Can you work these out from the model? Positions are in its coordinate system, mm. A direction names the side the tool comes from. Round coordinates to 2 decimals unless told otherwise and drop trailing zeros. Write each loop counter-clockwise with the first axis right and the second up, starting at its lowest first coordinate (ties: lowest second). Pieces come first, ordered by that corner, then holes. Notation, with made-up numbers: M 73.25,52.5 L 85.25,52.5 A19 cw 85.25,61.5 Z; hole C 75,2 d7. An arc over 180 degrees is marked long. Answer as a JSON object with one key per item and string values. Group by question number.
1) Suppose I cut it at B-B, the plane y = 3.05. Write out the boundary of the cut face in (x, z), and give its area (3 significant figures).
2) If we mould it in two halves opening along Z, with no side actions, what happens to faces 4 (the flat face through (21, 4, 24.95)), 5 (the flat face through (-44.95, 4, 0)), 6 (the cylindrical face through (-0.06, 1.02, -20.66))? For each: +Z half, -Z half, draft (parallel to the pull), parting line (faces both ways), or undercut.
3) On a 3-axis mill with a long thin cutter (end or side, diameter ignored), from which of +Z, -Z, +X, -X, +Y, -Y can I reach the whole of each face in a straight line? I mean faces 1 (the flat face through (2.65, 1.9, 25.1)), 2 (the flat face through (-38.59, 3.84, -24.126)), 3 (the flat face through (-3.5, 3.8, 24.1)). Say none if no direction works.
4) Suppose I cut it at C-C, the plane x = -27.5. Write out the boundary of the cut face in (y, z).
5) I'm going to push flat-ended pins straight in: pin 1 Ø1 at (y, z) = (3.5, 25.5) entering from -X; pin 2 Ø1 at (y, z) = (1.5, -25.5) entering from +X; pin 3 Ø2.5 at (y, z) = (3, 24.5) entering from -X; pin 4 Ø10 at (x, z) = (-10, 0.5) entering from -Y. Where does each tip first touch, or does it pass through?
6) Suppose I cut it at D-D, the plane x = 22. Write out the boundary of the cut face in (y, z).
7) Suppose I cut it at A-A, the plane z = -3. Write out the boundary of the cut face in (x, y), and give its area (3 significant figures).
8) Please list where these lines run through material, in increasing order: L1, parallel to X at y = 4.35, z = -1; L2, parallel to Z at x = 14, y = 4.6; L3, parallel to Z at x = -27, y = 4.7. Write a range as [from, to].
from build123d import *

# Parameters (mm, degrees)
CROQUIS1_W              = 92.4
CROQUIS1_H              = 52.4
SALIENTE_EXTRUIR1_DEPTH = 5
CROQUIS2_W              = 89.9
CROQUIS2_H              = 49.9
CORTAR_EXTRUIR1_DEPTH   = 2.93
CORTAR_EXTRUIR2_START   = -2.07
CORTAR_EXTRUIR2_DEPTH   = 5
CORTAR_EXTRUIR3_START   = -2.07
CORTAR_EXTRUIR3_DEPTH   = 5
SIMETR_A2_START         = -2.07
SIMETR_A2_COPY_1_DEPTH  = 5
SALIENTE_EXTRUIR3_START = -36.764169
SALIENTE_EXTRUIR3_DEPTH = 36.764169
CORTAR_EXTRUIR5_REACH   = 55.193


with BuildPart() as part:
    # Croquis1 → Saliente-Extruir1 (new body)
    with BuildSketch(Plane(origin=(0, 0, 0), x_dir=(1, 0, 0), z_dir=(0, 1, 0))):
        Rectangle(CROQUIS1_W, CROQUIS1_H)
    extrude(amount=SALIENTE_EXTRUIR1_DEPTH)

    # Croquis2 → Cortar-Extruir1 (cut)
    with BuildSketch(Plane(origin=(0, 5, 0), x_dir=(1, 0, 0), z_dir=(0, 1, 0))):
        Rectangle(CROQUIS2_W, CROQUIS2_H)
    extrude(amount=-CORTAR_EXTRUIR1_DEPTH, mode=Mode.SUBTRACT)

    # Croquis3 → Cortar-Extruir2 (cut)
    with BuildSketch(Plane(origin=(0, 2.07, 0), x_dir=(1, 0, 0), z_dir=(0, 1, 0)).offset(CORTAR_EXTRUIR2_START)):
        with BuildLine():
            Line((2.65, -23.31), (2.65, -26.2))
            Line((2.65, -26.2), (-2.65, -26.2))
            Line((-2.65, -26.2), (-2.65, -23.31))
            ThreePointArc((-2.65, -23.31), (0, -20.66), (2.65, -23.31))
        make_face()
    cortar_extruir2 = extrude(amount=CORTAR_EXTRUIR2_DEPTH, mode=Mode.SUBTRACT)

    # Croquis4 → Cortar-Extruir3 (cut)
    with BuildSketch(Plane(origin=(0, 2.07, 0), x_dir=(1, 0, 0), z_dir=(0, 1, 0)).offset(CORTAR_EXTRUIR3_START)):
        with BuildLine():
            Line((-46.2, -19.414169174), (-46.2, -26.2))
            Line((-46.2, -26.2), (-39.414169174, -26.2))
            Line((-39.414169174, -26.2), (-39.414169174, -24.95))
            ThreePointArc((-39.414169174, -24.95), (-41.32096321, -21.32096321), (-44.95, -19.414169174))
            Line((-44.95, -19.414169174), (-46.2, -19.414169174))
        make_face()
    cortar_extruir3 = extrude(amount=CORTAR_EXTRUIR3_DEPTH, mode=Mode.SUBTRACT)

    # Simetría1: Cortar-Extruir3 across plane
    add(cortar_extruir3.mirror(Plane(origin=(0, 0, 0), x_dir=(0, 0, 1), z_dir=(1, 0, 0))), mode=Mode.SUBTRACT)

    # Simetría2: Cortar-Extruir3 across plane
    add(cortar_extruir3.mirror(Plane.XY), mode=Mode.SUBTRACT)

    # Simetría2 copy 1 sketch → Simetría2 copy 1 (cut)
    with BuildSketch(Plane(origin=(0, 2.07, 0), x_dir=(-1, 0, 0), z_dir=(0, 1, 0)).offset(SIMETR_A2_START)):
        with BuildLine():
            Line((-46.2, -19.414169174), (-46.2, -26.2))
            Line((-46.2, -26.2), (-39.414169174, -26.2))
            Line((-39.414169174, -26.2), (-39.414169174, -24.95))
            ThreePointArc((-39.414169174, -24.95), (-41.32096321, -21.32096321), (-44.95, -19.414169174))
            Line((-44.95, -19.414169174), (-46.2, -19.414169174))
        make_face()
    extrude(amount=SIMETR_A2_COPY_1_DEPTH, mode=Mode.SUBTRACT)

    # Simetría3: Cortar-Extruir2 across plane
    add(cortar_extruir2.mirror(Plane.XY), mode=Mode.SUBTRACT)

    # Croquis7 → Saliente-Extruir3 (add)
    with BuildSketch(Plane(origin=(-2.65, 0, 0), x_dir=(0, 0, -1), z_dir=(1, 0, 0)).offset(SALIENTE_EXTRUIR3_START)):
        with BuildLine():
            Line((-24.95, 2.07), (-24.95, 5))
            Line((-24.95, 5), (-22.8, 5))
            ThreePointArc((-22.8, 5), (-22.523509792, 4.816418061), (-22.585410307, 4.490354433))
            Line((-22.585410307, 4.490354433), (-24.95, 2.07))
        make_face()
    saliente_extruir3 = extrude(amount=SALIENTE_EXTRUIR3_DEPTH)

    # Cortar-Extruir5: up to this face of the body (flat: up to its plane)
    cortar_extruir5_end = Plane(part.part.faces().sort_by_distance((21.032084587, 5, 25.575))[0])
    # Croquis8 → Cortar-Extruir5 (cut, up to the picked face)
    with BuildSketch(Plane(origin=(0, 2.07, 0), x_dir=(1, 0, 0), z_dir=(0, 1, 0)), mode=Mode.PRIVATE) as cortar_extruir5_sk1:
        with BuildLine():
            Line((-39.414169174, -24.95), (-37.257062393, -22.792893219))
            ThreePointArc((-37.257062393, -22.792893219), (-36.932639044, -22.576120467), (-36.549955612, -22.5))
            Line((-36.549955612, -22.5), (-5.514213562, -22.5))
            ThreePointArc((-5.514213562, -22.5), (-5.13153013, -22.576120467), (-4.807106781, -22.792893219))
            Line((-4.807106781, -22.792893219), (-2.65, -24.95))
            Line((-2.65, -24.95), (-1.683524182, -24.95))
            Line((-1.683524182, -24.95), (-1.683524182, -18.227572619))
            Line((-1.683524182, -18.227572619), (-40.735830346, -18.227572619))
            Line((-40.735830346, -18.227572619), (-40.735830346, -24.95))
            Line((-40.735830346, -24.95), (-39.414169174, -24.95))
        make_face()
    cortar_extruir5_tool1 = split(extrude(cortar_extruir5_sk1.sketch, amount=CORTAR_EXTRUIR5_REACH, mode=Mode.PRIVATE), bisect_by=cortar_extruir5_end, keep=Keep.BOTH, mode=Mode.PRIVATE)
    cortar_extruir5 = cortar_extruir5_tool1.solids().sort_by(Axis((-21.293277, 2.07, 20.569176), (0, 1, 0)))[0]
    add(cortar_extruir5, mode=Mode.SUBTRACT)

    # Simetría4: Saliente-Extruir3, Cortar-Extruir5 across plane
    add(saliente_extruir3.mirror(Plane.XY))
    add(cortar_extruir5.mirror(Plane.XY), mode=Mode.SUBTRACT)


solid = part.part
Results:
{
 "1": {"outline": "M -46.2,-19.41 L -44.95,-19.41 L -44.95,19.41 L -46.2,19.41 Z; M -39.41,-26.2 L -2.65,-26.2 L -2.65,-24.95 L -3.61,-23.99 L -38.46,-23.99 L -39.41,-24.95 Z; M -39.41,24.95 L -38.46,23.99 L -3.61,23.99 L -2.65,24.95 L -2.65,26.2 L -39.41,26.2 Z; M 2.65,-26.2 L 39.41,-26.2 L 39.41,-24.95 L 2.65,-24.95 Z; M 2.65,24.95 L 39.41,24.95 L 39.41,26.2 L 2.65,26.2 Z; M 44.95,-19.41 L 46.2,-19.41 L 46.2,19.41 L 44.95,19.41 Z", "area": "349 mm^2"},
 "2": {"face 4": "undercut", "face 5": "draft", "face 6": "-Z half"},
 "3": {"face 1": "+Z, +Y, -Y", "face 2": "-X, +Y", "face 3": "+X, +Y"},
 "4": {"outline": "M 0,-26.2 L 5,-26.2 L 5,-22.8 A0.3 ccw 4.49,-22.59 L 2.07,-24.95 L 2.07,24.95 L 4.49,22.59 A0.3 ccw 5,22.8 L 5,26.2 L 0,26.2 Z"},
 "5": {"pin 1": "x = -39.41", "pin 2": "x = 39.41", "pin 3": "x = -39.78", "pin 4": "y = 0"},
 "6": {"outline": "M 0,-26.2 L 5,-26.2 L 5,-24.95 L 2.07,-24.95 L 2.07,24.95 L 5,24.95 L 5,26.2 L 0,26.2 Z"},
 "7": {"outline": "M -46.2,0 L 46.2,0 L 46.2,5 L 44.95,5 L 44.95,2.07 L -44.95,2.07 L -44.95,5 L -46.2,5 Z", "area": "199 mm^2"},
 "8": {"L1": "[-46.2, -44.95], [44.95, 46.2]", "L2": "[-26.2, -24.95], [24.95, 26.2]", "L3": "[-26.2, -22.5], [22.5, 26.2]"}
}
